```python
from build123d import *

# Parameters (mm, degrees)
F0_W     = 40
F0_H     = 40
F1_DEPTH = 25


with BuildPart() as f1:
    # F0 (on Front) → F1 (new body)
    with BuildSketch(Plane.XZ):
        Polygon((-40, 75), (-45, 75), (-45, 0), (0, 0), (0, 75), align=None)
        with Locations((-20, 95)):
            Rectangle(F0_W, F0_H)
        Polygon((0, 0), (-45, 0), (-48, 0), (-48, -8), (0, -8), align=None)
        Polygon((0, -108), (0, -8), (-48, -8), (-50, -8), (-50, -108), align=None)
    extrude(amount=F1_DEPTH)


solid = f1.part
```
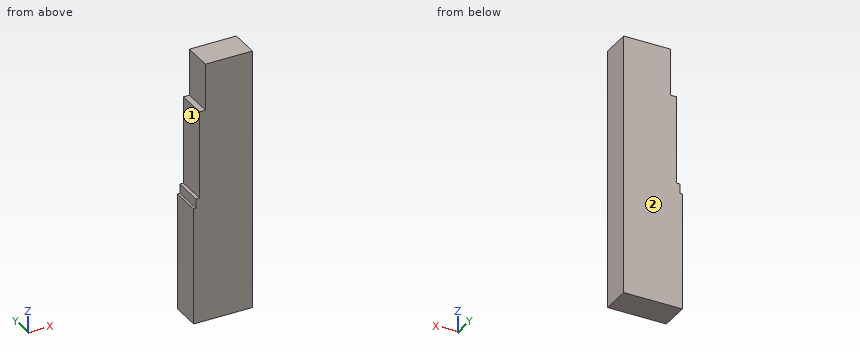
Can you work these out from the model? Positions are in its coordinate system, mm. Face numbers are marked on the shaded views. A direction names the side the tool comes from. Round coordinates to 2 decimals unless told otherwise and drop trailing zeros. Loops run counter-clockwise (first coordinate to the right, second up) from the corner with the lowest first, then second, coordinate; pieces in that order, holes last. Notation, with made-up numbers: M -17,10 L -7,10 A18 ccw -7,21 Z; hole C -5.5,-28.5 d5. An arc over 180 degrees is marked long. Answer in a Markdown table with one row per item.
1. If we section it at A-A, the plane y = -7: Please give me the cut outline in (x, z), plus the area to 3 significant figures.
Established:
| item | result |
|---|---|
| outline | M -50,-108 L 0,-108 L 0,115 L -40,115 L -40,75 L -45,75 L -45,0 L -48,0 L -48,-8 L -50,-8 Z |
| area | 10,400 mm² |
2. I'm going to push flat-ended pins straight in: pin 1 Ø6 at (y, z) = (-3, -2) entering from -X; pin 2 Ø3.5 at (x, y) = (-47, -18) entering from +Z; pin 3 Ø5 at (y, z) = (-19, 56.5) entering from +X; pin 4 Ø1.5 at (x, y) = (-42.5, -6.5) entering from +Z. Where does each tip first touch, or does it pass through?
Established:
| item | result |
|---|---|
| pin 1 | x = -48 |
| pin 2 | z = 0 |
| pin 3 | x = 0 |
| pin 4 | z = 75 |
3. If we section it at B-B, the plane z = 5.5: Please give me the cut outline in (x, y).
Established:
| item | result |
|---|---|
| outline | M -45,-25 L 0,-25 L 0,0 L -45,0 Z |
4. Please list where these lines run through material, in increasing order: line 1 (X direction, y = -11.5, z = 32.5); line 2 (Z direction, x = -44, y = -19); line 3 (X direction, y = -9, z = 90). Write a range as from..to.
Established:
| item | result |
|---|---|
| line 1 | -45..0 |
| line 2 | -108..75 |
| line 3 | -40..0 |
5. On a 3-axis mill with a long thin cutter (end or side, diameter ignored), from which of +Z, -Z, +X, -X, +Y, -Y can I reach the whole of each face in a straight line? I mean the marked faces 1 and 2. Say none if no direction works.
Established:
| item | result |
|---|---|
| face 1 | +Z, -X, +Y, -Y |
| face 2 | +Z, -Z, +X, -X, +Y |
